Answer from the drawing. Dimensions are ordinates in mm from the lowest x, y and z of the part. Give positions to 0.01 mm unless a question says otherwise; leave off trailing zeros. Loops run counter-clockwise (first coordinate to the right, second up) from the corner with the lowest first, then second, coordinate; pieces in that order, holes last. Notation, with made-up numbers: (38, -35.75) - (50, -35.75) arc R10 ccw to (50, -25.75) - close; hole circle Ø5 at (36.5, -37). An arc over 180 degrees is marked (long way). One line per item, written item: value.
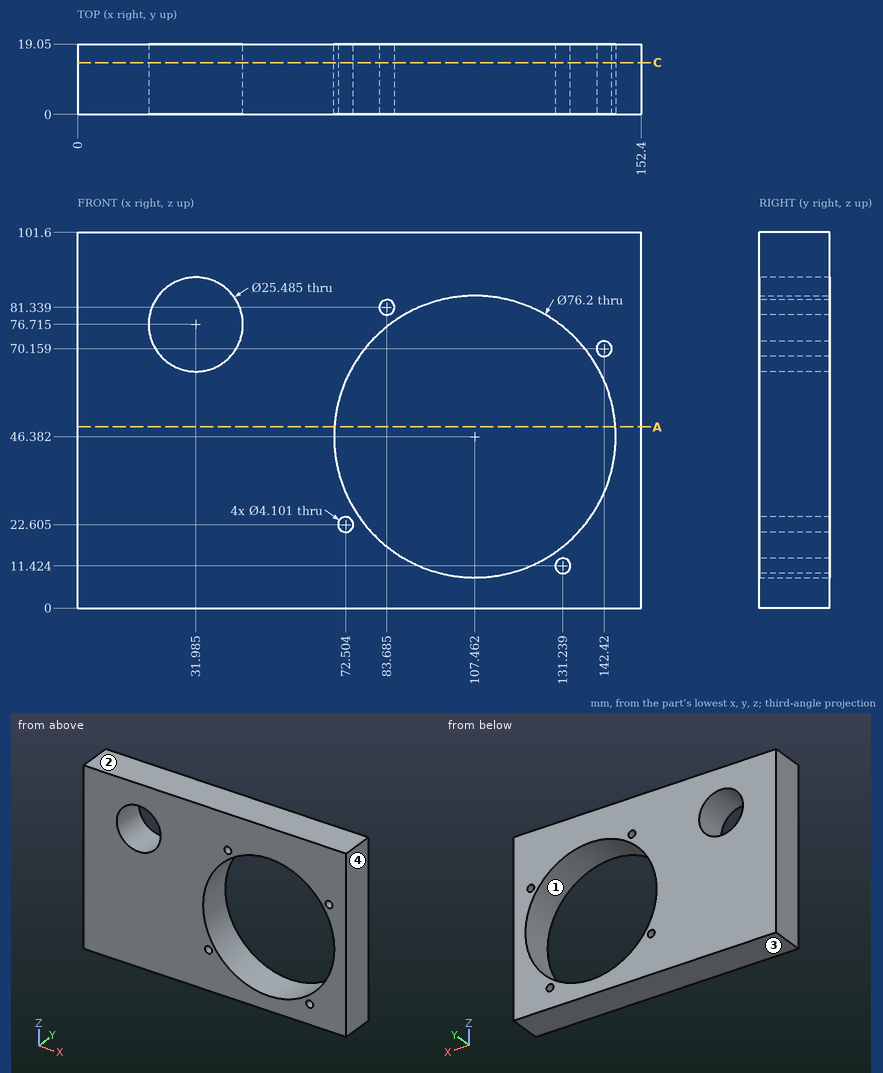
1. Section C-C (y = 14) is taken. Count the separate pieces of the cut face and the enclosed holes in it, and give its area (3 significant figures).
Output:
separate pieces: 1
enclosed holes: 6
area: 10,400 mm²
2. Section A-A (z = 49) is taken. Write down the section's boundary in (x, y).
Output:
outline: (0, 0) - (69.45, 0) - (69.45, 19.05) - (0, 19.05) - close; (145.47, 0) - (152.4, 0) - (152.4, 19.05) - (145.47, 19.05) - close
3. The mould has two halves that part along Z. Classify the marked faces 1, 2, 3 and 4: released by +Z, released by -Z, zero draft, split by the parting line, or undercut.
Output:
face 1: undercut
face 2: released by +Z
face 3: released by -Z
face 4: zero draft
4. Find the intervals of material crossed by line 1 along X through (y, z) = (7.75, 23) (1 decimal); line 2 along Z through (x, y) = (132, 5) (1 decimal); line 3 along X through (y, z) = (16.5, 68) (1 decimal), in increasing order.
Output:
line 1: x = 0 to 70.5, 74.5 to 77.4, 137.5 to 152.4
line 2: z = 0 to 9.5, 13.3 to 17.2, 75.5 to 101.6
line 3: x = 0 to 22.7, 41.3 to 76.1, 138.8 to 152.4
